from build123d import *

# Parameters (mm, degrees)
SKETCH2_W           = 127
SKETCH2_H           = 101.6
SKETCH2_W_2         = 101.6
SKETCH2_H_2         = 76.2
BOSS_EXTRUDE2_DEPTH = 914.4
SKETCH1_R           = 38.1
BOSS_EXTRUDE3_DEPTH = 44.45
BOSS_EXTRUDE5_START = -44.45
SKETCH3_R           = 38.1
BOSS_EXTRUDE5_DEPTH = 44.45
FILLET1_R           = 12.7
FILLET2_R           = 12.7


with BuildPart() as part:
    # Sketch2 → Boss-Extrude2 (new body)
    with BuildSketch(Plane.XY):
        with Locations((-63.5, 50.8)):
            Rectangle(SKETCH2_W, SKETCH2_H)
        with Locations((-63.5, 50.8)):
            Rectangle(SKETCH2_W_2, SKETCH2_H_2, mode=Mode.SUBTRACT)
    extrude(amount=BOSS_EXTRUDE2_DEPTH)

    # Sketch1 → Boss-Extrude3 (add)
    with BuildSketch(Plane(origin=(0, 0, 0), x_dir=(0, 0, -1), z_dir=(1, 0, 0))):
        with BuildLine():
            Line((-127, 101.6), (0, 101.6))
            Line((0, 101.6), (0, 304.8))
            ThreePointArc((0, 304.8), (-55.382017361, 361.922646449), (-114.190611982, 308.334272869))
            Line((-114.190611982, 308.334272869), (-127, 101.6))
        make_face()
        with Locations((-57.15, 304.8)):
            Circle(SKETCH1_R, mode=Mode.SUBTRACT)
    extrude(amount=-BOSS_EXTRUDE3_DEPTH)

    # Sketch3 → Boss-Extrude5 (add)
    with BuildSketch(Plane.ZY.offset(127).offset(BOSS_EXTRUDE5_START)):
        with BuildLine():
            Line((0, 304.8), (0, 101.6))
            Line((0, 101.6), (127, 101.6))
            Line((127, 101.6), (114.190611982, 308.334272869))
            ThreePointArc((114.190611982, 308.334272869), (55.382017361, 361.922646449), (0, 304.8))
        make_face()
        with Locations(Location((57.15, 304.8, 0), (0, 0, 180))):
            Circle(SKETCH3_R, mode=Mode.SUBTRACT)
    extrude(amount=BOSS_EXTRUDE5_DEPTH)

    # Fillet1
    fillet1_edges = [part.edges().sort_by_distance(p)[0] for p in [
        (-12.7, 88.9, 457.2),
        (-114.3, 88.9, 457.2),
        (-114.3, 12.7, 457.2),
        (-12.7, 12.7, 457.2),
    ]]
    fillet(fillet1_edges, radius=FILLET1_R)

    # Fillet2
    fillet2_edges = [part.edges().sort_by_distance(p)[0] for p in [
        (-44.45, 101.6, 63.5),
        (-22.225, 101.6, 127),
        (-82.55, 101.6, 63.5),
        (-104.775, 101.6, 127),
    ]]
    fillet(fillet2_edges, radius=FILLET2_R)


solid = part.part
Geometry: final body of the model. Coordinates: model frame, mm. A direction names the side the tool comes from. Coordinates: 2 decimals unless noted, no trailing zeros. Loops run counter-clockwise (first coordinate to the right, second up) from the corner with the lowest first, then second, coordinate; pieces in that order, holes last. Notation, with made-up numbers: (17.5, -38) - (39.5, -38) arc R14 ccw to (39.5, -26) - close; hole circle Ø10 at (27, -38.5). An arc over 180 degrees is marked (long way). Put each result on its own line as item: value. Start each with the question number.
Q1. Cut plane C-C, the plane y = 236. Return loops of the section in (x, z), and give its area (4 significant figures).
Q2. Pull-direction query (Z, two-part tool) for faces 4 (the flat face through (-64, 101.6, 451)), 5 (the flat face through (-21.93, 212.29, 120.14)), 6 (the cylindrical face through (-104.464, 327.983, 87.385)), 7 (the cylindrical face through (-21.914, 281.617, 87.385)); classes: released by +Z, released by -Z, zero draft, split by the parting line, or undercut.
Q3. Cut plane A-A, the plane z = 57.15. Return loops of the section in (x, y), and give its area (3 significant figures).
Q4. Cut plane B-B, the plane z = 184. Return loops of the section in (x, y), and give its area (3 significant figures).
Q5. Cut plane D-D, the plane y = 157. Return loops of the section in (x, z), and give its area (3 significant figures).
Q6. Line query: line 1 (Y direction, x = -24.5, z = 57.15); line 2 (Y direction, x = -25.5, z = 426); line 3 (Y direction, x = -113, z = 57.15). Output: solid intervals per line, ascending.
Q7. Set-up query: faces 1 (the flat face through (-44.45, 212, 64)), 2 (the flat face through (-64, 12.7, 451)), 3 (the cylindrical face through (-21.91, 361.87, 54.15)). Return all of +Z, -Z, +X, -X, +Y, -Y with unobstructed straight access to the full face (end or side cutting, diameter ignored); none if empty.
Filled sheet:
1. outline: (-127, 0) - (-82.55, 0) - (-82.55, 118.67) - (-127, 118.67) - close; (-44.45, 0) - (0, 0) - (0, 118.67) - (-44.45, 118.67) - close
1. area: 10,550 mm²
2. face 4: zero draft
2. face 5: released by +Z
2. face 6: undercut
2. face 7: undercut
3. outline: (-127, 0) - (0, 0) - (0, 266.7) - (-44.45, 266.7) - (-44.45, 114.3) arc R12.7 cw to (-57.15, 101.6) - (-69.85, 101.6) arc R12.7 cw to (-82.55, 114.3) - (-82.55, 266.7) - (-127, 266.7) - close; (-127, 342.9) - (-82.55, 342.9) - (-82.55, 361.95) - (-127, 361.95) - close; (-44.45, 342.9) - (0, 342.9) - (0, 361.95) - (-44.45, 361.95) - close; hole (-114.3, 25.4) arc R12.7 ccw to (-101.6, 12.7) - (-25.4, 12.7) arc R12.7 ccw to (-12.7, 25.4) - (-12.7, 76.2) arc R12.7 ccw to (-25.4, 88.9) - (-101.6, 88.9) arc R12.7 ccw to (-114.3, 76.2) - close
3. area: 21,700 mm²
4. outline: (-127, 0) - (0, 0) - (0, 101.6) - (-127, 101.6) - close; hole (-114.3, 25.4) arc R12.7 ccw to (-101.6, 12.7) - (-25.4, 12.7) arc R12.7 ccw to (-12.7, 25.4) - (-12.7, 76.2) arc R12.7 ccw to (-25.4, 88.9) - (-101.6, 88.9) arc R12.7 ccw to (-114.3, 76.2) - close
4. area: 5,300 mm²
5. outline: (-127, 0) - (-82.55, 0) - (-82.55, 123.57) - (-127, 123.57) - close; (-44.45, 0) - (0, 0) - (0, 123.57) - (-44.45, 123.57) - close
5. area: 11,000 mm²
6. line 1: 0 to 12.73, 88.87 to 266.7, 342.9 to 361.95
6. line 2: 0 to 12.7, 88.9 to 101.6
6. line 3: 0 to 19.8, 81.8 to 266.7, 342.9 to 361.95
7. face 1: +Z, -Z, +Y
7. face 2: +Z, -Z
7. face 3: +X, -X, +Y
